from build123d import *

# Parameters (mm, degrees)
SKETCH1_W           = 97.2
SKETCH1_H           = 26.25
BOSS_EXTRUDE1_DEPTH = 3
BOSS_EXTRUDE2_DEPTH = 22
SKETCH3_W           = 6.5
SKETCH3_H           = 20.25
CUT_EXTRUDE1_DEPTH  = 4
SKETCH5_R           = 1
CUT_EXTRUDE2_DEPTH  = 4
SKETCH6_W           = 55.45
SKETCH6_H           = 3
BOSS_EXTRUDE3_DEPTH = 3


with BuildPart() as part:
    # Sketch1 → Boss-Extrude1 (new body)
    with BuildSketch(Plane(origin=(0, 0, 0), x_dir=(1, 0, 0), z_dir=(0, 1, 0))):
        Rectangle(SKETCH1_W, SKETCH1_H)
    extrude(amount=BOSS_EXTRUDE1_DEPTH)

    # Sketch2 → Boss-Extrude2 (add)
    with BuildSketch(Plane(origin=(0, 3, 0), x_dir=(1, 0, 0), z_dir=(0, 1, 0))):
        Polygon((48.6, -13.125), (9.85, -13.125), (6.85, -13.125), (6.85, -7.125), (9.85, -7.125), (9.85, -10.125), (45.6, -10.125), (45.6, 10.125), (9.85, 10.125), (9.85, 7.125), (6.85, 7.125), (6.85, 13.125), (9.6, 13.125), (45.6, 13.125), (48.6, 13.125), align=None)
    extrude(amount=BOSS_EXTRUDE2_DEPTH)

    # Sketch3 → Cut-Extrude1 (cut, through all)
    with BuildSketch(Plane(origin=(0, 3, 0), x_dir=(1, 0, 0), z_dir=(0, 1, 0))):
        with Locations((17.6, 0)):
            Rectangle(SKETCH3_W, SKETCH3_H)
    extrude(amount=-CUT_EXTRUDE1_DEPTH, mode=Mode.SUBTRACT)

    # Sketch5 → Cut-Extrude2 (cut, through all)
    with BuildSketch(Plane(origin=(0, 3, 0), x_dir=(1, 0, 0), z_dir=(0, 1, 0))):
        with Locations((-32.1, 0)):
            Circle(SKETCH5_R)
        with Locations((-16.8, 0)):
            Circle(SKETCH5_R)
        with Locations((-13.7, 0)):
            Circle(SKETCH5_R)
        with Locations((-10.6, 0)):
            Circle(SKETCH5_R)
        with Locations((-7.5, 0)):
            Circle(SKETCH5_R)
        with Locations((-4.4, 0)):
            Circle(SKETCH5_R)
        with Locations((-35.2, 0)):
            Circle(SKETCH5_R)
        with Locations((-38.3, 0)):
            Circle(SKETCH5_R)
        with Locations((-41.4, 0)):
            Circle(SKETCH5_R)
        with Locations((-44.5, 0)):
            Circle(SKETCH5_R)
    extrude(amount=-CUT_EXTRUDE2_DEPTH, mode=Mode.SUBTRACT)

    # Sketch6 → Boss-Extrude3 (add)
    with BuildSketch(Plane(origin=(0, 3, 0), x_dir=(1, 0, 0), z_dir=(0, 1, 0))):
        with Locations((-20.875, 11.625)):
            Rectangle(SKETCH6_W, SKETCH6_H)
        with Locations((-20.875, -11.625)):
            Rectangle(SKETCH6_W, SKETCH6_H)
    extrude(amount=BOSS_EXTRUDE3_DEPTH)


solid = part.part
Source: CAD feature listing. Evaluate the final solid. Frame: model axes, mm. A direction names the side the tool comes from. Coordinates: 2 decimals unless noted, no trailing zeros. Loops run counter-clockwise (first coordinate to the right, second up) from the corner with the lowest first, then second, coordinate; pieces in that order, holes last. Notation, with made-up numbers: (76, 23) - (114, 23) arc R23 ccw to (114, 62) - close; hole circle Ø1 at (-32.5, -31.75). An arc over 180 degrees is marked (long way). Return JSON: item names as keys, results as strings.
Q1. Material intervals for line 1 along X through (y, z) = (6.25, 8); line 2 along Z through (x, y) = (10, 23) (3 decimals), sorted ascending.
Results:
{"line 1": "6.85 to 9.85, 45.6 to 48.6", "line 2": "-13.125 to -10.125, 10.125 to 13.125"}
Q2. Access query for faces 1 (the flat face through (21, 10, 13.125)), 2 (the flat face through (-21, 4, 10.125)), 3 (the flat face through (20.85, 2, 0)), 4 (the flat face through (31, 25, -11)), 5 (the flat face through (33, 3, 0)). Directions: +Z, -Z, +X, -X, +Y, -Y. A direction counts if a zero-diameter tool reaches every point of the face in a straight line with its end or side. Return the directions, or none.
Results:
{"face 1": "+Z, +X, -X, +Y, -Y", "face 2": "-X, +Y", "face 3": "+Y, -Y", "face 4": "+Z, -Z, +X, -X, +Y", "face 5": "+Y"}
Q3. Section A-A, the plane x = -44.5. Return loops of the section in (y, z) (3 decimals), plus the area to 4 significant figures.
Results:
{"outline": "(0, -13.125) - (6, -13.125) - (6, -10.125) - (3, -10.125) - (3, -1) - (0, -1) - close; (0, 1) - (3, 1) - (3, 10.125) - (6, 10.125) - (6, 13.125) - (0, 13.125) - close", "area": "90.75 mm2"}
Q4. Section B-B, the plane z = -8.75. Return loops of the section in (x, y).
Results:
{"outline": "(-48.6, 0) - (14.35, 0) - (14.35, 3) - (9.85, 3) - (9.85, 25) - (6.85, 25) - (6.85, 3) - (-48.6, 3) - close; (20.85, 0) - (48.6, 0) - (48.6, 25) - (45.6, 25) - (45.6, 3) - (20.85, 3) - close"}
Q5. Mould query, pull axis X, two halves, no side actions, for faces 6 (the cylindrical face through (-31.146, 1.521, -0.3)), 7 (the flat face through (-48.6, 2, 0)), 8 (the flat face through (-21, 4, -10.125)). Classes: released by +X, released by -X, zero draft, split by the parting line, or undercut.
Results:
{"face 6": "undercut", "face 7": "released by -X", "face 8": "zero draft"}
Q6. Contact query for flat-ended pins moving along their axis: P1, Ø2, axis at x = -23.5, z = -6.5, coming from the +Y side; P2, Ø3, axis at y = 18, z = 10, coming from the -X side; P3, Ø1.2, axis at x = -16.8, z = 0, coming from the +Y side; P4, Ø1, axis at y = 6, z = 1, coming from the -X side. Output: stop coordinate, or through.
Results:
{"P1": "y = 3", "P2": "x = 6.85", "P3": "through", "P4": "x = 45.6"}
Q7. Section C-C, the plane x = -26. Return loops of the section in (y, z) (3 decimals).
Results:
{"outline": "(0, -13.125) - (6, -13.125) - (6, -10.125) - (3, -10.125) - (3, 10.125) - (6, 10.125) - (6, 13.125) - (0, 13.125) - close"}
Q8. Section D-D, the plane y = 17. Return loops of the section in (x, z) (3 decimals), plus the area to 3 significant figures.
Results:
{"outline": "(6.85, -13.125) - (48.6, -13.125) - (48.6, 13.125) - (6.85, 13.125) - (6.85, 7.125) - (9.85, 7.125) - (9.85, 10.125) - (45.6, 10.125) - (45.6, -10.125) - (9.85, -10.125) - (9.85, -7.125) - (6.85, -7.125) - close", "area": "329 mm2"}
